Verification items for the finished model (mm, model axes). Coordinates: 2 decimals unless noted, no trailing zeros. Write each loop counter-clockwise with the first axis right and the second up, starting at its lowest first coordinate (ties: lowest second). Pieces come first, ordered by that corner, then holes. Notation, with made-up numbers: (-12, 52) - (-3, 52) arc R27 cw to (-3, 70) - close; hole circle Ø9 at (28, 44.5). An arc over 180 degrees is marked (long way). Use one line per item in the form item = value. Start each with the question number.
(1) Sectioned sample at A-A (y = 4). Record the cut outline in (x, z).
(2) Gauge pin test, flat end, axial feed: pin 1 Ø1.5 at (x, z) = (0, 93.5) entering from -Y. Record the tip position at first contact, or that the pin passes through.
(3) Sectioned sample at B-B (x = 0.95). Record the cut outline in (y, z).
(4) Material ranges on line 1 (Z direction, x = 1.2, y = 15); line 2 (Z direction, x = -1, y = 4.5); line 3 (Y direction, x = -1.15, z = 129), recorded low to high. Write a range as [from, to].
Autodesk Inventor part; units mm, degrees
ref_plane "YZ Plane" through (0, 0, 0) normal (1, 0, 0) x (0, 1, 0)
ref_plane "XZ Plane" through (0, 0, 0) normal (0, 1, 0) x (-1, 0, 0)
ref_plane "XY Plane" through (0, 0, 0) normal (0, 0, 1) x (1, 0, 0)
sketch "Sketch2" plane through (0, 0, 0) normal (0, 1, 0) x (-1, 0, 0)
  line L0 (-1.5, -198.6195) -> (1.5, -198.6195)
  line L1 (1.5, -198.6195) -> (1.5, 198.6195)
  line L2 (1.5, 198.6195) -> (-1.5, 198.6195)
  line L3 (-1.5, 198.6195) -> (-1.5, -198.6195)
  line L4 (-1.5, -198.6195) -> (1.5, 198.6195) construction
  line L5 (1.5, -198.6195) -> (-1.5, 198.6195) construction
  point P0 (0, 0)
  dimension "d0" = 3
  dimension "d1" = 397.239
extrude "Extrusion1" add sketch "Sketch2" along normal blind 30
sketch "Sketch3" plane through (1.5, 0, 198.6195) normal (1, 0, 0) x (0, 0, -1)
  line L0 (397.239, 0) -> (0, 0)
  line L1 (68, 0) -> (82, 0)
  line L2 (82, 0) -> (82, 14)
  line L3 (68, 14) -> (68, 0)
  arc A0 (82, 14) -> (68, 14) centre (75, 14) ccw
  arc A1 (68, 14) -> (82, 14) centre (75, 14) ccw construction
  line L4 (0, 0) -> (0, 30)
  point P0 (198.6195, 0)
  dimension "d4" = 14
  dimension "d5" = 14
  dimension "d6" = 14
  dimension "d9" = 75
extrude "Extrusion2" cut sketch "Sketch3" against normal through all
sketch "Sketch4" plane through (1.5, 0, -198.6195) normal (1, 0, 0) x (0, 0, -1)
  line L0 (-329.239, 0) -> (-397.239, 0)
  line L1 (-397.239, 0) -> (-397.239, 30)
  line L2 (-397.239, 0) -> (-397.239, 30)
  line L3 (-397.239, 30) -> (-391.9492, 30)
  line L4 (-397.239, 30) -> (0, 30)
  line L5 (-397.239, 0) -> (-391.9492, 30)
  point P0 (-198.6195, 0)
  dimension "d10" = 10
extrude "Extrusion3" cut sketch "Sketch4" against normal through all
properties part number "wall-inner-plunger"
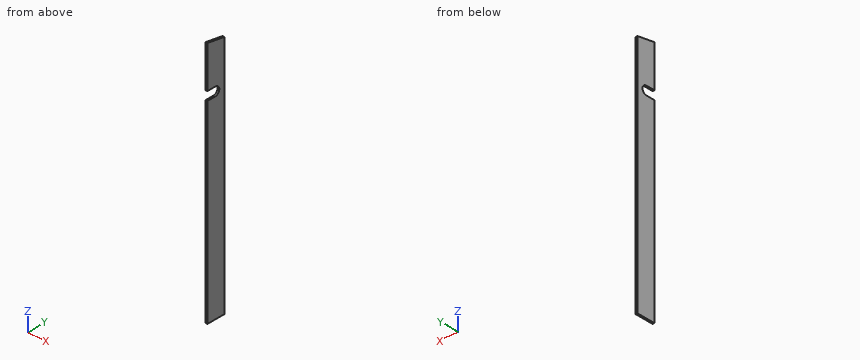
Answers below:
q1.outline = (-1.5, -198.62) - (1.5, -198.62) - (1.5, 116.62) - (-1.5, 116.62) - close; (-1.5, 130.62) - (1.5, 130.62) - (1.5, 197.91) - (-1.5, 197.91) - close
q2.pin_1 = 0
q3.outline = (0, -198.62) - (30, -198.62) - (30, 193.33) - (0, 198.62) - (0, 130.62) - (14, 130.62) arc R7 cw to (14, 116.62) - (0, 116.62) - close
q4.line_1 = [-198.62, 116.69], [130.55, 195.97]
q4.line_2 = [-198.62, 116.62], [130.62, 197.83]
q4.line_3 = [18.48, 30]
